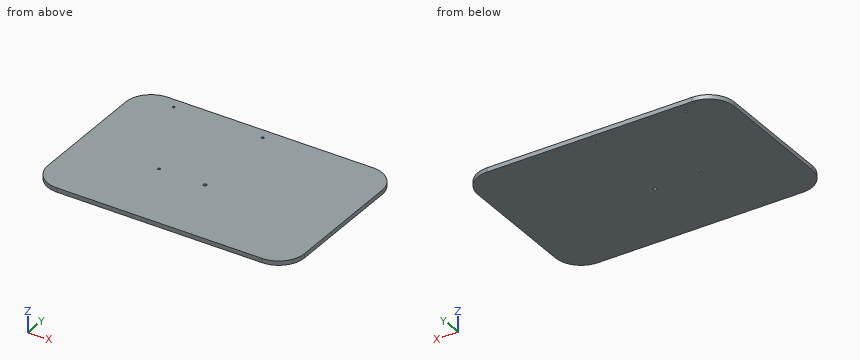
```python
from build123d import *

# Parameters (mm, degrees)
SALIENTE_EXTRUIR1_DEPTH = 5
CROQUIS2_R              = 1.465459125
CROQUIS2_R_2            = 2
CORTAR_EXTRUIR1_DEPTH   = 5


with BuildPart() as part:
    # Croquis1 → Saliente-Extruir1 (new body)
    with BuildSketch(Plane.XY):
        with BuildLine():
            Line((30, 0), (270, 0))
            ThreePointArc((270, 0), (291.213203436, 8.786796564), (300, 30))
            Line((300, 30), (300, 170))
            ThreePointArc((300, 170), (291.213203436, 191.213203436), (270, 200))
            Line((270, 200), (30, 200))
            ThreePointArc((30, 200), (8.786796564, 191.213203436), (0, 170))
            Line((0, 170), (0, 30))
            ThreePointArc((0, 30), (8.786796564, 8.786796564), (30, 0))
        make_face()
    extrude(amount=SALIENTE_EXTRUIR1_DEPTH)

    # Croquis2 → Cortar-Extruir1 (cut)
    with BuildSketch(Plane(origin=(0, 0, 0), x_dir=(-1, 0, 0), z_dir=(0, 0, -1))):
        with Locations((-148.851699579, 187.841418575)):
            Circle(CROQUIS2_R)
        with Locations((-44.851699579, 187.841418575)):
            Circle(CROQUIS2_R)
        with Locations((-94.851699579, 83.841418575)):
            Circle(CROQUIS2_R)
        with Locations((-148.851699579, 83.841418575)):
            Circle(CROQUIS2_R_2)
    extrude(amount=-CORTAR_EXTRUIR1_DEPTH, mode=Mode.SUBTRACT)


solid = part.part
```
Read the model definition and answer for the solid it produces. Units are mm, in the model's axes. Give positions to 0.01 mm unless a question says otherwise; leave off trailing zeros. Order: outer loops, then holes, each group sorted by start corner. A loop starts at its lowest first (then second) coordinate and runs counter-clockwise, first axis right, second up. Notation, with made-up numbers: (-38, 44) -> (16, 44) arc R18 ccw to (16, 77) -> close; hole circle Ø8 at (-30.5, 50.25). An arc over 180 degrees is marked (long way). One line per item, written item: value. Start each with the question number.
(1) The part is cut by section A-A (x = 281.5). Determine the outline of the cut face in (y, z).
(2) Flat-ended cylindrical pins translate along their axes: P1, Ø3, axis at x = 148.85, y = 83.84, coming from the -Z side; P2, Ø12, axis at x = 52.5, y = 99, coming from the -Z side. Find the tip coordinate at first contact, or state that the pin passes through.
(3) Straight lines are drawn through the part: L1, parallel to Y at x = 95, z = 1.9; L2, parallel to Y at x = 285.5, z = 0.9; L3, parallel to X at y = 13.5, z = 0.7. For each, find the intervals that lie inside material, in ascending order.
Taken from the geometry:
1. outline: (2.29, 0) -> (197.71, 0) -> (197.71, 5) -> (2.29, 5) -> close
2. P1: through
2. P2: z = 0
3. L1: 0 to 82.38, 85.3 to 200
3. L2: 4.31 to 195.69
3. L3: 4.95 to 295.05
